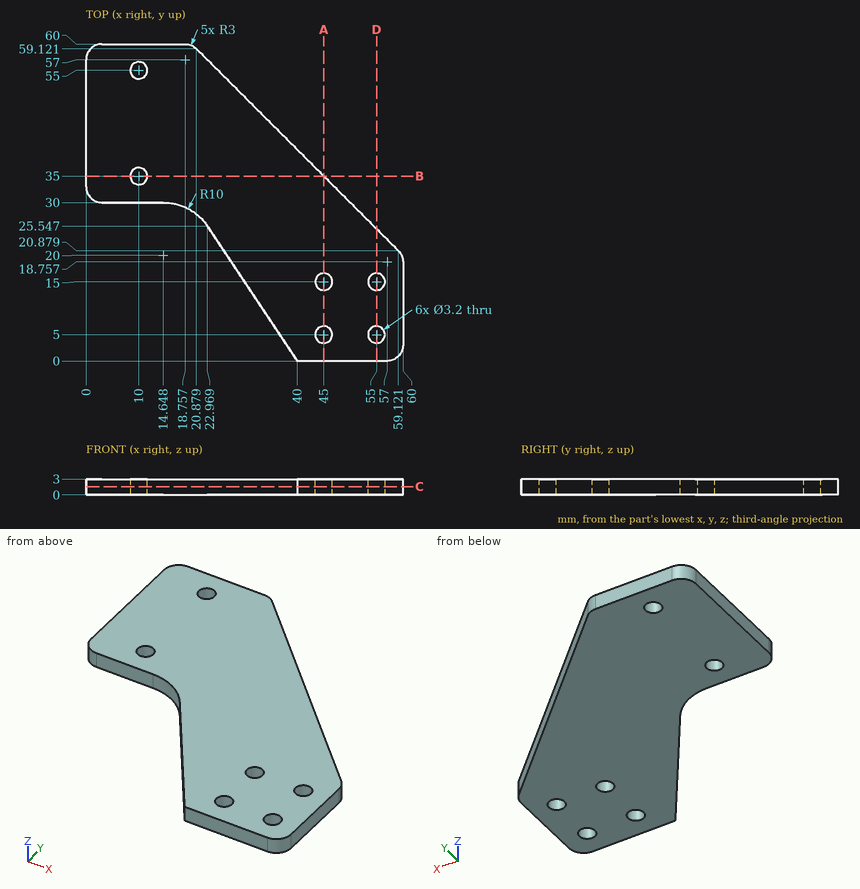
Can you work these out from the drawing? Everything is in mm from the part's minimum corner. Coordinates: 2 decimals unless noted, no trailing zeros. Loops run counter-clockwise (first coordinate to the right, second up) from the corner with the lowest first, then second, coordinate; pieces in that order, holes last.
1) Imagine slicing it at B-B on y = 35. List the corners of the cut face in (x, z) for me, plus the area to 3 significant figures.
2) Imagine slicing it at D-D on x = 55. List the corners of the cut face in (y, z) for me.
3) For pin 1 (5 mm diameter, centred on x = 10, y = 35, fed in from +Z); pin 2 (1.5 mm diameter, centred on y = 18.5, z = 0.5, fed in from -X); pin 3 (1.5 mm diameter, centred on y = 19.5, z = 2, fed in from -X), each with a flat end and sliding along its axis, tell me the tip position at first contact or that it passes through.
4) I need wall thicknesses on probe 1 along Y at (x, z) = (10, 1.25); probe 2 along Y at (x, z) = (55, 1); probe 3 along Y at (x, z) = (13.5, 1.05). Which ranges of each line are inside material? Lowest first, please.
5) Imagine slicing it at C-C on z = 1.55. List the corners of the cut face in (x, y) for me.
6) Imagine slicing it at A-A on x = 45. List the corners of the cut face in (y, z) for me.
Completed:
1. outline: (0, 0) - (8.4, 0) - (8.4, 3) - (0, 3) - close; (11.6, 0) - (45, 0) - (45, 3) - (11.6, 3) - close
1. area: 125 mm2
2. outline: (0, 0) - (3.4, 0) - (3.4, 3) - (0, 3) - close; (6.6, 0) - (13.4, 0) - (13.4, 3) - (6.6, 3) - close; (16.6, 0) - (25, 0) - (25, 3) - (16.6, 3) - close
3. pin 1: stops at z = 3
3. pin 2: stops at x = 27.17
3. pin 3: stops at x = 26.5
4. probe 1: y = 30 to 33.4, 36.6 to 53.4, 56.6 to 60
4. probe 2: y = 0 to 3.4, 6.6 to 13.4, 16.6 to 25
4. probe 3: y = 30 to 60
5. outline: (0, 33) arc R3 ccw to (3, 30) - (14.65, 30) arc R10 cw to (22.97, 25.55) - (40, 0) - (57, 0) arc R3 ccw to (60, 3) - (60, 18.76) arc R3 ccw to (59.12, 20.88) - (20.88, 59.12) arc R3 ccw to (18.76, 60) - (3, 60) arc R3 ccw to (0, 57) - close; hole circle Ø3.2 at (10, 35); hole circle Ø3.2 at (10, 55); hole circle Ø3.2 at (45, 5); hole circle Ø3.2 at (45, 15); hole circle Ø3.2 at (55, 5); hole circle Ø3.2 at (55, 15)
6. outline: (0, 0) - (3.4, 0) - (3.4, 3) - (0, 3) - close; (6.6, 0) - (13.4, 0) - (13.4, 3) - (6.6, 3) - close; (16.6, 0) - (35, 0) - (35, 3) - (16.6, 3) - close
